Model file for the job. Use its own axes, mm. A direction names the side the tool comes from. Coordinates: 2 decimals unless noted, no trailing zeros. Order: outer loops, then holes, each group sorted by start corner. A loop starts at its lowest first (then second) coordinate and runs counter-clockwise, first axis right, second up. Notation, with made-up numbers: (3, 74.5) -> (37, 74.5) arc R23 ccw to (37, 100.5) -> close; hole circle Ø10 at (65.25, 41.25). An arc over 180 degrees is marked (long way). Return JSON: item names as keys, results as strings. Group by question number.
1) Cut at D-D (x = -2.5). Write the cut outline in (y, z).
2) Pull direction Y, two halves, no side cores. Call faces 1 (the flat face through (0, -5, -20)), 2 (the cylindrical face through (-224.93, -46.553, 17.692)), 3 (the flat face through (-101.68, -32.365, 0.07)): +Y half, -Y half, draft (parallel to the pull), parting line (faces both ways), or undercut.
3) Probe line 1 (Z direction, x = -178, y = -4.5); line 2 (Z direction, x = -15, y = -6.75); line 3 (Y direction, x = -55.5, z = 16.5). List the from-to ranges inside material, lowest first.
4) Which spindle directions (+Z, -Z, +X, -X, +Y, -Y) get a long thin tool onto all of the face, cutting with end or side? Do faces 4 (the flat face through (-91, -10, 23)), 5 (the cylindrical face through (-224.93, -12.44, 20.12)), 6 (the flat face through (-118.6, -4.93, 21.906)). Say none if no direction does.
5) Flat gauge pins, fed straight in: pin 1 (19.5 mm diameter, centred on y = -40, z = -24, fed in from +X); pin 2 (11 mm diameter, centred on x = 2.5, y = -5.5, fed in from +Z); pin 3 (3 mm diameter, centred on x = -181, y = -24, fed in from -Z). Where does each tip first touch, or does it go through?
6) Cut at A-A (x = -103). Write the cut outline in (y, z).
7) Cut at C-C (x = -67). Write the cut outline in (y, z).
8) Cut at B-B (y = -49). Write the cut outline in (x, z), and give its area (3 significant figures).
Autodesk Inventor part; units mm, degrees
ref_plane "Work Plane1" through (-220, 0, 5) normal (0, 0, 1) x (1, 0, 0)
ref_plane "YZ Plane" through (0, 0, 0) normal (1, 0, 0) x (0, 1, 0)
ref_plane "XZ Plane" through (0, 0, 0) normal (0, 1, 0) x (-1, 0, 0)
sketch "Sketch1" plane through (0, 0, 0) normal (0, 1, 0) x (-1, 0, 0)
  line L0 (20, 20) -> (-20, 20)
  line L1 (-20, 20) -> (-20, -20)
  line L2 (-20, -20) -> (20, -20)
  line L3 (20, -20) -> (20, 20)
  line L4 (20, 20) -> (-20, -20) construction
  line L5 (-20, 20) -> (20, -20) construction
  line L6 (-20, 0) -> (230, 0)
  line L7 (230, 0) -> (230, 44.15)
  line L8 (230, 44.15) -> (220, 44.15)
  line L9 (220, 44.15) -> (230, 44.15)
  line L10 (230, 44.15) -> (230, -44.15)
  line L11 (230, -44.15) -> (220, -44.15)
  line L12 (220, -44.15) -> (220, 44.15)
  line L13 (220, 44.15) -> (20, 20)
  line L14 (220, -44.15) -> (20, -20)
  line L15 (20, -20) -> (20, -10)
  line L16 (20, 20) -> (20, 10)
  line L17 (220, 44.15) -> (220, 34.15)
  line L18 (220, -44.15) -> (220, -34.15)
  line L19 (20, 10) -> (220, 34.15)
  line L20 (220, -34.15) -> (20, -10)
  line L21 (220, 0) -> (220, -5)
  line L22 (20, 0) -> (20, 5)
  line L23 (220, -5) -> (20, -5)
  line L24 (20, -5) -> (20, 5)
  line L25 (20, 5) -> (220, 5)
  line L26 (220, 5) -> (220, -5)
  line L27 (-20, 20) -> (-20, 15)
  line L28 (-20, 15) -> (-15, 15)
  line L29 (20, -20) -> (15, -20)
  line L30 (15, -20) -> (15, -15)
  circle A0 centre (15, -15) radius 1.5
  circle A1 centre (-15, 15) radius 1.5
  point P0 (0, 0)
  dimension "d0" = 40
  dimension "d1" = 40
  dimension "d2" = 250
  dimension "d3" = 44.15
  dimension "d4" = 10
  dimension "d5" = 88.3
  dimension "d6" = 10
  dimension "d7" = 10
  dimension "d8" = 10
  dimension "d9" = 10
  dimension "d10" = 5
  dimension "d11" = 5
  dimension "d12" = 5
  dimension "d13" = 5
  dimension "d14" = 3
  dimension "d15" = 3
extrude "Extrusion1" add sketch "Sketch1" against normal blind 10 contours L3 L6 L1 L0 | L13 L12 L19 L3 | L8 L7 L6 L12 | L25 L12 L6 L3 | L6 L3 L2 L1 | L6 L12 L23 L3 | L10 L11 L12 L6 | L20 L12 L14 L3
sketch "Sketch2" plane through (0, -10, 0) normal (0, -1, 0) x (1, 0, 0)
  line L0 (-230, 44.15) -> (-230, -44.15)
  line L1 (-230, 44.15) -> (-220, 44.15)
  line L2 (-230, -44.15) -> (-220, -44.15)
  line L3 (-220, -44.15) -> (-220, 44.15)
  line L4 (-220, 44.15) -> (-230, 44.15)
  line L5 (-230, 44.15) -> (-230, -44.15)
  point P0 (0, 0)
extrude "Extrusion2" add sketch "Sketch2" along normal blind 44.112
ref_plane "Work Plane1" through (-220, 0, 5) normal (0, 0, 1) x (1, 0, 0)
sketch "Sketch3" plane through (-220, 0, 5) normal (0, 0, 1) x (1, 0, 0)
  line L0 (0, -10) -> (0, -54.112)
  line L1 (200, -10) -> (240, -10)
  line L2 (0, -54.112) -> (240, -10)
  line L3 (0, 0) -> (0, -10)
  line L4 (0, -54.112) -> (0, -10)
  line L5 (0, -10) -> (240, -10)
  point P0 (220, 0)
extrude "Extrusion3" add sketch "Sketch3" against normal blind 10
sketch "Sketch5" plane through (-220, 0, 34.15) normal (1, 0, 0) x (0, 0, -1)
  line L0 (0, 0) -> (29.15, 0)
  line L1 (0, 0) -> (14.575, 0)
  line L2 (14.575, 0) -> (14.575, -10)
  circle A0 centre (14.575, -10) radius 2.5
  line L3 (34.15, 0) -> (34.15, -54.112)
  line L4 (39.15, -54.112) -> (29.15, -54.112)
  circle A1 centre (53.725, -10) radius 2.5
  dimension "d23" = 14.575
  dimension "d24" = 10
  dimension "d25" = 5
extrude "Extrusion4" cut sketch "Sketch5" against normal blind 10
sketch "Sketch6" plane through (-220, 0, 34.15) normal (1, 0, 0) x (0, 0, -1)
  line L0 (-10, 0) -> (-10, -54.112)
  line L1 (-10, -54.112) -> (17, -54.112)
  line L2 (17, -54.112) -> (17, -44.112)
  circle A0 centre (17, -44.112) radius 2.5
  line L3 (34.15, 0) -> (34.15, -54.112)
  line L4 (39.15, -54.112) -> (29.15, -54.112)
  circle A1 centre (51.3, -44.112) radius 2.5
  dimension "d28" = 27
  dimension "d29" = 10
  dimension "d30" = 5
extrude "Extrusion5" cut sketch "Sketch6" against normal blind 10
properties part number "magnetometer_holder" material "PET Plastic"
Answers below:
{
 "1": {"outline": "(-14.14, -5) -> (-10, -5) -> (-10, -20) -> (0, -20) -> (0, 20) -> (-10, 20) -> (-10, 5) -> (-14.14, 5) -> close"},
 "2": {"face 1": "draft", "face 2": "undercut", "face 3": "-Y half"},
 "3": {"line 1": "z = -39.08 to -29.08, -5 to 5, 29.08 to 39.08", "line 2": "z = -20 to -16.5, -13.5 to 20", "line 3": "y = -10 to 0"},
 "4": {"face 4": "+Z, +X, -Y", "face 5": "-X", "face 6": "+Y, -Y"},
 "5": {"pin 1": "stops at x = -220", "pin 2": "stops at z = 20", "pin 3": "stops at z = -5"},
 "6": {"outline": "(-32.61, -5) -> (0, -5) -> (0, 5) -> (-32.61, 5) -> close; (-10, -30.02) -> (0, -30.02) -> (0, -20.02) -> (-10, -20.02) -> close; (-10, 20.02) -> (0, 20.02) -> (0, 30.02) -> (-10, 30.02) -> close"},
 "7": {"outline": "(-25.99, -5) -> (0, -5) -> (0, 5) -> (-25.99, 5) -> close; (-10, -25.68) -> (0, -25.68) -> (0, -15.68) -> (-10, -15.68) -> close; (-10, 15.68) -> (0, 15.68) -> (0, 25.68) -> (-10, 25.68) -> close"},
 "8": {"outline": "(-230, -44.15) -> (-220, -44.15) -> (-220, -5) -> (-192.19, -5) -> (-192.19, 5) -> (-220, 5) -> (-220, 44.15) -> (-230, 44.15) -> close", "area": "1,160 mm^2"}
}
